Check sheet for the modelled part. Datum: model origin and axes. Units: mm. Face numbers are marked on the shaded views. A direction names the side the tool comes from. Give positions to 0.01 mm unless a question says otherwise; leave off trailing zeros. Write each loop counter-clockwise with the first axis right and the second up, starting at its lowest first coordinate (ties: lowest second). Pieces come first, ordered by that corner, then holes. Notation, with made-up numbers: (77.25, 25) -> (91.25, 25) arc R9 cw to (91.25, 38) -> close; hole circle Ø11 at (25, 21). An arc over 180 degrees is marked (long way). Answer as a JSON object with one key per item and string values.
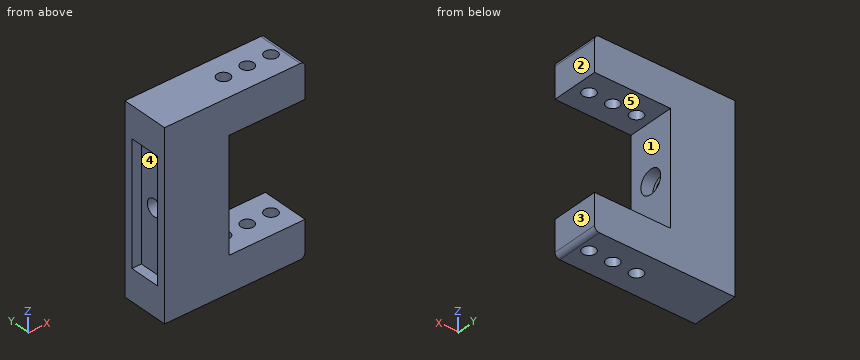
Autodesk Inventor part; units mm, degrees
ref_plane "YZ Plane" through (0, 0, 0) normal (1, 0, 0) x (0, 1, 0)
ref_plane "XZ Plane" through (0, 0, 0) normal (0, 1, 0) x (-1, 0, 0)
ref_plane "XY Plane" through (0, 0, 0) normal (0, 0, 1) x (1, 0, 0)
sketch "Boceto1" plane through (0, 0, 0) normal (0, 1, 0) x (-1, 0, 0)
  line L0 (-38.575, 38.575) -> (38.575, 38.575)
  line L1 (38.575, 38.575) -> (38.575, -38.575)
  line L2 (38.575, -38.575) -> (-38.575, -38.575)
  line L3 (-38.575, -38.575) -> (-38.575, 38.575)
  line L4 (-38.575, 38.575) -> (38.575, -38.575) construction
  line L5 (38.575, 38.575) -> (-38.575, -38.575) construction
  circle A0 centre (17, 10) radius 2.7
  circle A1 centre (17, -10) radius 2.7
  circle A2 centre (-17, -10) radius 2.7
  circle A3 centre (-17, 10) radius 2.7
  point P0 (0, 0)
  dimension "d0" = 77.15
  dimension "d1" = 77.15
  dimension "d2" = 5.4
  dimension "d3" = 10
  dimension "d4" = 10
  dimension "d5" = 17
  dimension "d6" = 17
extrude "Extrusión1" add sketch "Boceto1" along normal blind 20
sketch "Boceto2" plane through (0, 20, 0) normal (0, 1, 0) x (1, 0, 0)
  line L0 (-38.575, -38.575) -> (38.575, -38.575)
  line L1 (38.575, -38.575) -> (70.575, -38.575)
  line L2 (70.575, -38.575) -> (70.575, -23.575)
  line L3 (70.575, -23.575) -> (38.575, -23.575)
  line L4 (38.575, -23.575) -> (38.575, -38.575)
  line L5 (38.575, 38.575) -> (-38.575, 38.575)
  line L6 (38.575, 38.575) -> (70.575, 38.575)
  line L7 (70.575, 38.575) -> (70.575, 23.575)
  line L8 (70.575, 23.575) -> (38.575, 23.575)
  line L9 (38.575, 23.575) -> (38.575, 38.575)
  point P0 (0, 0)
  dimension "d9" = 32
  dimension "d10" = 15
extrude "Extrusión2" add sketch "Boceto2" against normal up to surface (20 mm away)
sketch "Boceto3" plane through (-38.575, 0, 38.575) normal (0, 0, 1) x (1, 0, 0)
  circle A0 centre (103.15, 10) radius 2.7
  circle A1 centre (93.15, 10) radius 2.7
  line L0 (109.15, 20) -> (109.15, 0)
  circle A2 centre (83.15, 10) radius 2.7
  point P0 (38.575, 0)
  dimension "d13" = 5.4
  dimension "d14" = 6
  dimension "d15" = 10
  dimension "d34" = 10
extrude "Extrusión3" cut sketch "Boceto3" against normal through all
fillet "Empalme2" radius 4.635 2 edges at (-38.575, 10, 38.575) (-38.575, 10, -38.575)
fillet "Empalme3" radius 2 2 edges at (70.575, 10, -38.575) (70.575, 10, 38.575)
sketch "Boceto5" plane through (0, 20, 0) normal (0, 1, 0) x (1, 0, 0)
  line L0 (-29.2306, -22.0337) -> (29.2306, -22.0337)
  line L1 (29.2306, -22.0337) -> (29.2306, 22.0337)
  line L2 (29.2306, 22.0337) -> (-29.2306, 22.0337)
  line L3 (-29.2306, 22.0337) -> (-29.2306, -22.0337)
  line L4 (-29.2306, -22.0337) -> (29.2306, 22.0337) construction
  line L5 (29.2306, -22.0337) -> (-29.2306, 22.0337) construction
  point P0 (0, 0)
extrude "Extrusión5" add sketch "Boceto5" against normal up to surface (20 mm away)
sketch "Boceto6" plane through (-38.575, 0, -33.94) normal (-1, 0, 0) x (0, 0, 1)
  line L0 (-23.6354, 28.4555) -> (91.5154, 28.4555)
  line L1 (91.5154, 28.4555) -> (91.5154, -11.4044)
  line L2 (91.5154, -11.4044) -> (-23.6354, -11.4044)
  line L3 (-23.6354, -11.4044) -> (-23.6354, 28.4555)
  line L4 (-23.6354, 28.4555) -> (91.5154, -11.4044) construction
  line L5 (91.5154, 28.4555) -> (-23.6354, -11.4044) construction
  point P0 (33.94, 0)
  point P1 (33.94, 8.5256)
extrude "Extrusión6" cut sketch "Boceto6" against normal blind 50
sketch "Boceto7" plane through (11.425, 0, -33.94) normal (-1, 0, 0) x (0, 0, 1)
  line L0 (59.44, 3.5) -> (8.44, 3.5)
  line L1 (8.44, 3.5) -> (8.44, 16.5)
  line L2 (8.44, 16.5) -> (59.44, 16.5)
  line L3 (59.44, 16.5) -> (59.44, 3.5)
  line L4 (59.44, 3.5) -> (8.44, 16.5) construction
  line L5 (8.44, 3.5) -> (59.44, 16.5) construction
  line L6 (72.515, 0) -> (-4.635, 0)
  point P0 (33.94, 0)
  point P1 (33.94, 10)
  point P2 (33.94, 10)
  point P3 (33.94, 0)
  dimension "d39" = 13
  dimension "d40" = 51
  dimension "d41" = 3.5
extrude "Extrusión7" cut sketch "Boceto7" against normal blind 4
sketch "Boceto8" plane through (15.425, 0, -33.94) normal (-1, 0, 0) x (0, 0, 1)
  circle A0 centre (33.94, 10) radius 3.5
  point P0 (33.94, 0)
  dimension "d44" = 7
extrude "Extrusión8" cut sketch "Boceto8" against normal through all
sketch "Boceto9" plane through (38.575, 0, 23.575) normal (1, 0, 0) x (0, 0, -1)
  circle A0 centre (23.575, 10) radius 3.5
  circle A1 centre (23.575, 10) radius 5
  point P0 (23.575, 0)
  dimension "d47" = 10
extrude "Extrusión9" cut sketch "Boceto9" against normal blind 5 contours A0 | A1
sketch "Boceto4" plane through (0, 20, 0) normal (0, 1, 0) x (1, 0, 0)
  line L0 (53.225, -32.695) -> (61.325, -32.695)
  line L1 (61.325, -32.695) -> (61.325, -28.455)
  line L2 (61.325, -28.455) -> (53.225, -28.455)
  line L3 (53.225, -28.455) -> (53.225, -32.695)
  line L4 (53.225, -32.695) -> (61.325, -28.455) construction
  line L5 (61.325, -32.695) -> (53.225, -28.455) construction
  line L6 (57.275, -38.575) -> (51.875, -38.575)
  point P0 (0, 0)
  point P1 (57.275, -30.575)
  dimension "d21" = 8.1
  dimension "d23" = 1.35
  dimension "d24" = 8
  dimension "d25" = 4.24
properties part number "LowerJawLoadCell" material "Plástico ABS"
1. Sectioned sample at A-A, the plane z = 26.5. Enter the section's corners in (x, y) (3 decimals), plus the area to 3 significant figures.
Determined:
{"outline": "(11.425, 0) -> (70.575, 0) -> (70.575, 20) -> (11.425, 20) -> close; hole circle Ø5.4 at (44.575, 10); hole circle Ø5.4 at (54.575, 10); hole circle Ø5.4 at (64.575, 10)", "area": "1,110 mm^2"}
2. Sectioned sample at C-C, the plane z = 0. Enter the section's corners in (x, y) (3 decimals), plus the area to 3 significant figures.
Determined:
{"outline": "(11.425, 0) -> (38.575, 0) -> (38.575, 5) -> (33.575, 5) -> (33.575, 6.5) -> (15.425, 6.5) -> (15.425, 3.5) -> (11.425, 3.5) -> close; (11.425, 16.5) -> (15.425, 16.5) -> (15.425, 13.5) -> (33.575, 13.5) -> (33.575, 15) -> (38.575, 15) -> (38.575, 20) -> (11.425, 20) -> close", "area": "314 mm^2"}
3. Sectioned sample at B-B, the plane x = 36. Enter the section's corners in (y, z) (3 decimals).
Determined:
{"outline": "(0, -38.575) -> (20, -38.575) -> (20, 38.575) -> (0, 38.575) -> close; hole circle Ø10 at (10, 0)"}
4. Go/stop test with flat-tipped pins: P1, Ø2, axis at x = 14, z = -1, coming from the -Y side; P2, Ø5, axis at x = 44.575, y = 10, coming from the +Z side; P3, Ø6.5, axis at y = 8.5, z = -4.5, coming from the -X side (3 decimals); P4, Ø11, axis at y = 11.5, z = 0, coming from the +X side (3 decimals). Record where each tip stops, or that it passes through.
Determined:
{"P1": "y = 0", "P2": "through", "P3": "x = 15.425", "P4": "x = 38.575"}
5. Mould release check, pull along X, two halves, no side actions. Record for the marked faces 3, 4 and 5: released by +X, released by -X, zero draft, split by the parting line, or undercut.
Determined:
{"face 3": "released by +X", "face 4": "released by -X", "face 5": "zero draft"}
6. Sectioned sample at D-D, the plane x = 56. Enter the section's corners in (y, z) (3 decimals).
Determined:
{"outline": "(0, -38.575) -> (7.707, -38.575) -> (7.707, -23.575) -> (0, -23.575) -> close; (0, 23.575) -> (7.707, 23.575) -> (7.707, 38.575) -> (0, 38.575) -> close; (12.293, -38.575) -> (20, -38.575) -> (20, -23.575) -> (12.293, -23.575) -> close; (12.293, 23.575) -> (20, 23.575) -> (20, 38.575) -> (12.293, 38.575) -> close"}
7. Scan lines: L1, parallel to Z at x = 43, y = 18.25 (3 decimals); L2, parallel to Y at x = 35.65, z = 0; L3, parallel to Z at x = 15, y = 7.75 (3 decimals). Record each from-to range of solid material in increasing order. Write a range as [from, to].
Determined:
{"L1": "[-38.575, -23.575], [23.575, 38.575]", "L2": "[0, 5], [15, 20]", "L3": "[-38.575, -25.5], [25.5, 38.575]"}
8. Access from +Z, -Z, +X, -X, +Y, -Y to the whole of each face (thin tool, end or side, straight path). Record for the marked faces 1 and 2.
Determined:
{"face 1": "+X, +Y, -Y", "face 2": "+Z, -Z, +X, +Y, -Y"}
